```python
from build123d import *

# Parameters (mm, degrees)
SKETCH1_W                                      = 203.2
SKETCH1_H                                      = 177
BOSS_EXTRUDE1_DEPTH                            = 0.6096
CUT_EXTRUDE7_DEPTH                             = 313.185220041
SKETCH4_W                                      = 196.85
SKETCH4_H                                      = 0.6096
BOSS_EXTRUDE2_DEPTH                            = 12
SKETCH14_W                                     = 196.85
SKETCH14_H                                     = 11.938
BOSS_EXTRUDE3_DEPTH                            = 0.6096
SKETCH13_W                                     = 196.85
SKETCH13_H                                     = 0.6096
CUT_EXTRUDE9_DEPTH                             = 12
CSK_FOR_M3_FLAT_HEAD_MACHINE_SCREW3_AT_2_COUNT = 2
CSK_FOR_M3_FLAT_HEAD_MACHINE_SCREW3_AT_2_PITCH = 25
CSK_FOR_M3_FLAT_HEAD_MACHINE_SCREW3_AT_3_COUNT = 2
CSK_FOR_M3_FLAT_HEAD_MACHINE_SCREW3_AT_3_PITCH = 50
CSK_FOR_M3_FLAT_HEAD_MACHINE_SCREW3_AT_4_COUNT = 2
CSK_FOR_M3_FLAT_HEAD_MACHINE_SCREW3_AT_4_PITCH = 75
CSK_FOR_M3_FLAT_HEAD_MACHINE_SCREW3_AT_5_COUNT = 2
CSK_FOR_M3_FLAT_HEAD_MACHINE_SCREW3_AT_5_PITCH = 100
CSK_FOR_M3_FLAT_HEAD_MACHINE_SCREW3_AT_6_COUNT = 2
CSK_FOR_M3_FLAT_HEAD_MACHINE_SCREW3_AT_6_PITCH = 125
CSK_FOR_M3_FLAT_HEAD_MACHINE_SCREW3_AT_7_COUNT = 2
CSK_FOR_M3_FLAT_HEAD_MACHINE_SCREW3_AT_7_PITCH = 150


with BuildPart() as part:
    # Sketch1 → Boss-Extrude1 (new body)
    with BuildSketch(Plane(origin=(0, 0, 0), x_dir=(1, 0, 0), z_dir=(0, 0, -1))):
        with Locations((-101.6, 148.5)):
            Rectangle(SKETCH1_W, SKETCH1_H)
    extrude(amount=BOSS_EXTRUDE1_DEPTH)

    # Sketch2 → Cut-Extrude7 (cut, through all)
    with BuildSketch(Plane(origin=(0, 0, -0.6096), x_dir=(1, 0, 0), z_dir=(0, 0, -1))):
        with BuildLine():
            Line((-131.7, 173.5), (-131.7, 148))
            ThreePointArc((-131.7, 148), (-138.2, 141.5), (-144.7, 148))
            Line((-144.7, 148), (-144.7, 173.5))
            ThreePointArc((-144.7, 173.5), (-138.2, 180), (-131.7, 173.5))
        make_face()
        with BuildLine():
            Line((-58.5, 173.5), (-58.5, 148))
            ThreePointArc((-58.5, 148), (-65, 141.5), (-71.5, 148))
            Line((-71.5, 148), (-71.5, 173.5))
            ThreePointArc((-71.5, 173.5), (-65, 180), (-58.5, 173.5))
        make_face()
    extrude(amount=-CUT_EXTRUDE7_DEPTH, mode=Mode.SUBTRACT)

    # Sketch4 → Boss-Extrude2 (add)
    with BuildSketch(Plane.XY):
        with Locations((-101.6, -60.3048)):
            Rectangle(SKETCH4_W, SKETCH4_H)
    extrude(amount=BOSS_EXTRUDE2_DEPTH)

    # Sketch14 → Boss-Extrude3 (add)
    with BuildSketch(Plane.XY):
        with Locations((-101.6, -54.031)):
            Rectangle(SKETCH14_W, SKETCH14_H)
    extrude(amount=-BOSS_EXTRUDE3_DEPTH)

    # Sketch13 → Cut-Extrude9 (cut)
    with BuildSketch(Plane.XY.offset(12)):
        with Locations((-101.6, -60.3048)):
            Rectangle(SKETCH13_W, SKETCH13_H)
    extrude(amount=-CUT_EXTRUDE9_DEPTH, mode=Mode.SUBTRACT)

    # Sketch16 → CSK for M3 Flat Head Machine Screw3 (revolve, cut)
    with BuildSketch(Plane(origin=(-185.47, -222, 0), x_dir=(0, -1, 0), z_dir=(1, 0, 0))):
        Polygon((0, 0), (0, 0.6096), (1.7, 0.6096), (1.7, 2.15), (3.85, 0), align=None)
    csk_for_m3_flat_head_machine_screw3 = revolve(axis=Axis((-185.47, -222, 6.35), (0, 0, -1)), mode=Mode.SUBTRACT)

    # CSK for M3 Flat Head Machine Screw3 at 2: CSK for M3 Flat Head Machine Screw3 ×2
    with Locations(*[(0, i * CSK_FOR_M3_FLAT_HEAD_MACHINE_SCREW3_AT_2_PITCH, 0) for i in range(1, CSK_FOR_M3_FLAT_HEAD_MACHINE_SCREW3_AT_2_COUNT)]):
        add(csk_for_m3_flat_head_machine_screw3, mode=Mode.SUBTRACT)

    # CSK for M3 Flat Head Machine Screw3 at 3: CSK for M3 Flat Head Machine Screw3 ×2
    with Locations(*[(0, i * CSK_FOR_M3_FLAT_HEAD_MACHINE_SCREW3_AT_3_PITCH, 0) for i in range(1, CSK_FOR_M3_FLAT_HEAD_MACHINE_SCREW3_AT_3_COUNT)]):
        add(csk_for_m3_flat_head_machine_screw3, mode=Mode.SUBTRACT)

    # CSK for M3 Flat Head Machine Screw3 at 4: CSK for M3 Flat Head Machine Screw3 ×2
    with Locations(*[(0, i * CSK_FOR_M3_FLAT_HEAD_MACHINE_SCREW3_AT_4_PITCH, 0) for i in range(1, CSK_FOR_M3_FLAT_HEAD_MACHINE_SCREW3_AT_4_COUNT)]):
        add(csk_for_m3_flat_head_machine_screw3, mode=Mode.SUBTRACT)

    # CSK for M3 Flat Head Machine Screw3 at 5: CSK for M3 Flat Head Machine Screw3 ×2
    with Locations(*[(0, i * CSK_FOR_M3_FLAT_HEAD_MACHINE_SCREW3_AT_5_PITCH, 0) for i in range(1, CSK_FOR_M3_FLAT_HEAD_MACHINE_SCREW3_AT_5_COUNT)]):
        add(csk_for_m3_flat_head_machine_screw3, mode=Mode.SUBTRACT)

    # CSK for M3 Flat Head Machine Screw3 at 6: CSK for M3 Flat Head Machine Screw3 ×2
    with Locations(*[(0, i * CSK_FOR_M3_FLAT_HEAD_MACHINE_SCREW3_AT_6_PITCH, 0) for i in range(1, CSK_FOR_M3_FLAT_HEAD_MACHINE_SCREW3_AT_6_COUNT)]):
        add(csk_for_m3_flat_head_machine_screw3, mode=Mode.SUBTRACT)

    # CSK for M3 Flat Head Machine Screw3 at 7: CSK for M3 Flat Head Machine Screw3 ×2
    with Locations(*[(0, i * CSK_FOR_M3_FLAT_HEAD_MACHINE_SCREW3_AT_7_PITCH, 0) for i in range(1, CSK_FOR_M3_FLAT_HEAD_MACHINE_SCREW3_AT_7_COUNT)]):
        add(csk_for_m3_flat_head_machine_screw3, mode=Mode.SUBTRACT)

    # Mirror1: CSK for M3 Flat Head Machine Screw3 across plane
    add(csk_for_m3_flat_head_machine_screw3.mirror(Plane.ZY.offset(101.599999995)), mode=Mode.SUBTRACT)

    # Mirror1 copy 1 sketch → Mirror1 copy 1 (revolve, cut)
    with BuildSketch(Plane(origin=(-17.729999998, -197.000000003, 0), x_dir=(-3.839898042745385e-11, -1.0, 0), z_dir=(-1.0, 3.839898042745385e-11, 0))):
        Polygon((0, 0), (0, -0.6096), (1.7, -0.6096), (1.7, -2.15), (3.85, 0), align=None)
    revolve(axis=Axis((-17.729999998, -197.000000003, 6.35), (0, 0, 1)), mode=Mode.SUBTRACT)

    # Mirror1 copy 2 sketch → Mirror1 copy 2 (revolve, cut)
    with BuildSketch(Plane(origin=(-17.729999998, -172.000000003, 0), x_dir=(-3.839898042745385e-11, -1.0, 0), z_dir=(-1.0, 3.839898042745385e-11, 0))):
        Polygon((0, 0), (0, -0.6096), (1.7, -0.6096), (1.7, -2.15), (3.85, 0), align=None)
    revolve(axis=Axis((-17.729999998, -172.000000003, 6.35), (0, 0, 1)), mode=Mode.SUBTRACT)

    # Mirror1 copy 3 sketch → Mirror1 copy 3 (revolve, cut)
    with BuildSketch(Plane(origin=(-17.729999997, -147.000000003, 0), x_dir=(-3.839898042745385e-11, -1.0, 0), z_dir=(-1.0, 3.839898042745385e-11, 0))):
        Polygon((0, 0), (0, -0.6096), (1.7, -0.6096), (1.7, -2.15), (3.85, 0), align=None)
    revolve(axis=Axis((-17.729999997, -147.000000003, 6.35), (0, 0, 1)), mode=Mode.SUBTRACT)

    # Mirror1 copy 4 sketch → Mirror1 copy 4 (revolve, cut)
    with BuildSketch(Plane(origin=(-17.729999996, -122.000000003, 0), x_dir=(-3.839898042745385e-11, -1.0, 0), z_dir=(-1.0, 3.839898042745385e-11, 0))):
        Polygon((0, 0), (0, -0.6096), (1.7, -0.6096), (1.7, -2.15), (3.85, 0), align=None)
    revolve(axis=Axis((-17.729999996, -122.000000003, 6.35), (0, 0, 1)), mode=Mode.SUBTRACT)

    # Mirror1 copy 5 sketch → Mirror1 copy 5 (revolve, cut)
    with BuildSketch(Plane(origin=(-17.729999995, -97.000000003, 0), x_dir=(-3.839898042745385e-11, -1.0, 0), z_dir=(-1.0, 3.839898042745385e-11, 0))):
        Polygon((0, 0), (0, -0.6096), (1.7, -0.6096), (1.7, -2.15), (3.85, 0), align=None)
    revolve(axis=Axis((-17.729999995, -97.000000003, 6.35), (0, 0, 1)), mode=Mode.SUBTRACT)

    # Mirror1 copy 6 sketch → Mirror1 copy 6 (revolve, cut)
    with BuildSketch(Plane(origin=(-17.729999994, -72.000000003, 0), x_dir=(-3.839898042745385e-11, -1.0, 0), z_dir=(-1.0, 3.839898042745385e-11, 0))):
        Polygon((0, 0), (0, -0.6096), (1.7, -0.6096), (1.7, -2.15), (3.85, 0), align=None)
    revolve(axis=Axis((-17.729999994, -72.000000003, 6.35), (0, 0, 1)), mode=Mode.SUBTRACT)


solid = part.part
```
Can you work these out from the model? Positions are in its coordinate system, mm. Give positions to 0.01 mm unless a question says otherwise; leave off trailing zeros. Write each loop counter-clockwise with the first axis right and the second up, starting at its lowest first coordinate (ties: lowest second). Pieces come first, ordered by that corner, then holes. Notation, with made-up numbers: (29, 65.25) - (75, 65.25) arc R9 cw to (75, 75.25) - close; hole circle Ø3 at (4.5, -9). An arc over 180 degrees is marked (long way). Write item = value, one per line. Start each with the question number.
1. Please list where these lines run through material, in increasing order: line 1 (X direction, y = -158.5, z = -0.35); line 2 (X direction, y = -219, z = -0.1); line 3 (Y direction, x = -59, z = -0.4).
2. Thinking about a two-plate mould opening in Y: for faces 1 (the face through (-103, -141, 0)), 2 (the face through (-65.1, -180, -0.3)), which applies, released by +Y, released by -Y, zero draft, split by the parting line, or undercut?
3. Imagine slicing it at B-B (y = -163). Please give me the cut outline in (x, z).
4. Imagine slicing it at C-C (x = -65). Please give me the cut outline in (y, z).
5. Imagine slicing it at A-A (z = -0.25). Count the separate pieces of the cut face and the enclosed holes in it, and give its area (3 significant figures).
Worked answers:
q1.line_1 = -203.2 to -144.7, -131.7 to -71.5, -58.5 to 0
q1.line_2 = -203.2 to -187.72, -183.22 to -19.98, -15.48 to 0
q1.line_3 = -237 to -176, -145.5 to -48.06
q2.face_1 = zero draft
q2.face_2 = undercut
q3.outline = (-203.2, -0.61) - (-144.7, -0.61) - (-144.7, 0) - (-203.2, 0) - close; (-131.7, -0.61) - (-71.5, -0.61) - (-71.5, 0) - (-131.7, 0) - close; (-58.5, -0.61) - (0, -0.61) - (0, 0) - (-58.5, 0) - close
q4.outline = (-237, -0.61) - (-180, -0.61) - (-180, 0) - (-237, 0) - close; (-141.5, -0.61) - (-48.06, -0.61) - (-48.06, 0) - (-141.5, 0) - close
q5.separate_pieces = 1
q5.enclosed_holes = 16
q5.area = 36,800 mm2
